```python
from build123d import *

# Parameters (mm, degrees)
F1_DEPTH    = 12.7
F2_R        = 2.54
F3_R        = 1.27
F4_T1_DEPTH = 12.7


# Not quite as in the source:
# - a fillet or chamfer that OpenCascade refuses, or shapes differently, is made with other operations: its cross-section is extruded or revolved along the edge and cut away or added


with BuildPart() as f1:
    # F0 (on Front) → F1 (new body)
    with BuildSketch(Plane.XZ):
        Polygon((-29.21, 0), (0, 0), (0, 8.128), (-6.858, 8.128), (-6.8540549837, 4.3214331381), (-7.62, 4.3214331381), (-7.62, 9.906), (-29.21, 9.906), align=None)
    extrude(amount=F1_DEPTH)

    # F2
    f2_edges = [f1.edges().sort_by_distance(p)[0] for p in [
        (-29.21, -6.35, 9.906),
    ]]
    fillet(f2_edges, radius=F2_R)

    # F3
    f3_edges = [f1.edges().sort_by_distance(p)[0] for p in [
        (-7.62, -6.35, 9.906),
    ]]
    fillet(f3_edges, radius=F3_R)

    # F4: fillet of radius 1.016 on 1 edges, made by hand

    # F4_s2 → F4_t1 (join)
    with BuildSketch(Plane.XZ):
        with BuildLine():
            ThreePointArc((-7.62, 5.306181078), (-7.4059700317, 4.6824022163), (-6.8540549837, 4.3214331381))
            Line((-6.8540549837, 4.3214331381), (-7.62, 4.3214331381))
            Line((-7.62, 4.3214331381), (-7.62, 5.306181078))
        make_face()
    extrude(amount=F4_T1_DEPTH)

    # F5: F1 across face


with BuildPart() as f1_1:
    add(f1.part)
    add(f1.part.mirror(Plane(origin=(-14.605, -6.35, 0), x_dir=(1, 0, 0), z_dir=(0, 0, -1))))

    # F6: F1 across face


with BuildPart() as f1_2:
    add(f1_1.part)
    add(f1_1.part.mirror(Plane(origin=(0, -6.35, 0), x_dir=(0, 1, 0), z_dir=(1, 0, 0))))


solid = f1_2.part
```
Can you work these out from the model? Positions are in its coordinate system, mm. A direction names the side the tool comes from. Give positions to 0.01 mm unless a question says otherwise; leave off trailing zeros. Loops run counter-clockwise (first coordinate to the right, second up) from the corner with the lowest first, then second, coordinate; pieces in that order, holes last. Notation, with made-up numbers: M 43.5,-11 L 93.5,-11 A18 cw 93.5,15 Z; hole C -12.75,-25.5 d3. An arc over 180 degrees is marked long. One line per question, with ' | ' between items. Start each with the question number.
Q1. For faces 1 (the cylindrical face through (-8, -6.44, -9.54)), 2 (the flat face through (-7.62, -6, 7)), 3 (the cylindrical face through (28.45, -6.44, -9.18)), which set-ups out of +Z, -Z, +X, -X, +Y, -Y let a thin tool reach every point of the face, with its end or its side?
Q2. If we section it at B-B (z = -6): Please give me the cut outline in (x, y), plus the area to 3 significant figures.
Q3. If we mould it in two halves opening along Z, with no side actions, what happens to faces 4 (the flat face through (7.62, -6, 7)), 5 (the cylindrical face through (-28.45, -6.44, -9.18)), 6 (the flat face through (-18, -6, 9.906))? For each: +Z half, -Z half, draft (parallel to the pull), parting line (faces both ways), or undercut.
Q4. If we section it at C-C (x = -1.5): Please give me the cut outline in (y, z).
Q5. If I drill on line 1 (X direction, y = -8.5, z = -4.5); line 2 (X direction, y = -5.5, z = 5); line 3 (Z direction, x = -3, y = -11), over which ranges is the centre line in solid material (lowest first)? Write a range as from..to.
Q6. If we section it at A-A (y = -4.75): Please give me the cut outline in (x, z), plus the area to 3 significant figures.
Q7. For pin 1 Ø4 at (x, y) = (3, -7.5) entering from +Z, with a flat end and sliding along its axis, tell me the tip position at first contact or that it passes through.
Computed:
1) face 1: -Z, +Y, -Y | face 2: +Z, +Y, -Y | face 3: -Z, +X, +Y, -Y
2) outline: M -29.21,-12.7 L -7.62,-12.7 L -7.62,0 L -29.21,0 Z; M -6.86,-12.7 L 6.86,-12.7 L 6.86,0 L -6.86,0 Z; M 7.62,-12.7 L 29.21,-12.7 L 29.21,0 L 7.62,0 Z | area: 723 mm²
3) face 4: draft | face 5: -Z half | face 6: +Z half
4) outline: M -12.7,-8.13 L 0,-8.13 L 0,8.13 L -12.7,8.13 Z
5) line 1: x = -29.21..-7.22, -6.85..6.85, 7.22..29.21 | line 2: x = -29.21..-7.57, -6.85..6.85, 7.57..29.21 | line 3: z = -8.13..8.13
6) outline: M -29.21,-7.37 A2.54 ccw -26.67,-9.91 L -8.89,-9.91 A1.27 ccw -7.62,-8.64 L -7.62,-5.31 A1.02 cw -6.85,-4.32 L -6.86,-8.13 L 6.86,-8.13 L 6.85,-4.32 A1.02 cw 7.62,-5.31 L 7.62,-8.64 A1.27 ccw 8.89,-9.91 L 26.67,-9.91 A2.54 ccw 29.21,-7.37 L 29.21,7.37 A2.54 ccw 26.67,9.91 L 8.89,9.91 A1.27 ccw 7.62,8.64 L 7.62,5.31 A1.02 cw 6.85,4.32 L 6.86,8.13 L -6.86,8.13 L -6.85,4.32 A1.02 cw -7.62,5.31 L -7.62,8.64 A1.27 ccw -8.89,9.91 L -26.67,9.91 A2.54 ccw -29.21,7.37 Z | area: 1,090 mm²
7) pin 1: stops at z = 8.13
